Geometry: final body of the model. Coordinates: model frame, mm. A direction names the side the tool comes from. Give positions to 0.01 mm unless a question says otherwise; leave off trailing zeros. Write each loop counter-clockwise with the first axis right and the second up, starting at its lowest first coordinate (ties: lowest second). Pieces come first, ordered by that corner, then holes.
from build123d import *

# Parameters (mm, degrees)
SKETCH1_W           = 29.21
SKETCH1_H           = 35.56
SKETCH1_R           = 1.5499969
BOSS_EXTRUDE1_DEPTH = 5.08
SKETCH2_W           = 5.08
SKETCH2_H           = 25.4
SKETCH2_W_2         = 19.05
SKETCH2_H_2         = 5.08
CUT_EXTRUDE1_DEPTH  = 3.81


with BuildPart() as part:
    # Sketch1 → Boss-Extrude1 (new body)
    with BuildSketch(Plane(origin=(0, 0, 0), x_dir=(1, 0, 0), z_dir=(0, 1, 0))):
        with Locations((2.211294118, -3.505162647)):
            Rectangle(SKETCH1_W, SKETCH1_H)
        with Locations(Location((-9.788707282, 11.694832353, 0), (0, 0, 270))):
            Circle(SKETCH1_R, mode=Mode.SUBTRACT)
        with Locations(Location((14.211295518, 11.694832353, 0), (0, 0, 270))):
            Circle(SKETCH1_R, mode=Mode.SUBTRACT)
        with Locations(Location((14.211295518, -18.705157647, 0), (0, 0, 270))):
            Circle(SKETCH1_R, mode=Mode.SUBTRACT)
        with Locations(Location((-9.788707282, -18.705157647, 0), (0, 0, 270))):
            Circle(SKETCH1_R, mode=Mode.SUBTRACT)
    extrude(amount=BOSS_EXTRUDE1_DEPTH)

    # Sketch2 → Cut-Extrude1 (cut)
    with BuildSketch(Plane(origin=(0, 5.08, 0), x_dir=(1, 0, 0), z_dir=(0, 1, 0))):
        with Locations((-9.853705882, -3.505162647)):
            Rectangle(SKETCH2_W, SKETCH2_H)
        with Locations((2.211294118, 11.734837353)):
            Rectangle(SKETCH2_W_2, SKETCH2_H_2)
        with Locations((14.276294118, -3.505162647)):
            Rectangle(SKETCH2_W, SKETCH2_H)
        with Locations((2.211294118, -3.505162647)):
            Rectangle(SKETCH2_W_2, SKETCH2_H)
        with Locations((2.211294118, -18.745162647)):
            Rectangle(SKETCH2_W_2, SKETCH2_H_2)
    extrude(amount=-CUT_EXTRUDE1_DEPTH, mode=Mode.SUBTRACT)


solid = part.part
Q1. Section D-D on y = 0.5. Output: boundary loops of the cut face in (x, z), plus the area to 3 significant figures.
Filled sheet:
outline: (-12.39, -14.27) - (16.82, -14.27) - (16.82, 21.29) - (-12.39, 21.29) - close; hole circle Ø3.1 at (-9.79, -11.69); hole circle Ø3.1 at (-9.79, 18.71); hole circle Ø3.1 at (14.21, -11.69); hole circle Ø3.1 at (14.21, 18.71)
area: 1,010 mm2
Q2. Pull-direction query (Z, two-part tool) for faces 1 (the cylindrical face through (-9.323, 2.504, 20.184)), 2 (the flat face through (2, 1, -14.275)), 3 (the flat face through (2, 1, 21.285)); classes: released by +Z, released by -Z, zero draft, split by the parting line, or undercut.
Filled sheet:
face 1: undercut
face 2: released by -Z
face 3: released by +Z
Q3. Ray query, line 1 along X through (y, z) = (4.7, 17); line 2 along Z through (x, y) = (-8, 2.85); line 3 along Y through (x, z) = (2.75, -2). Return the intervals inside material, ascending.
Filled sheet:
line 1: x = -12.39 to -7.31, 11.74 to 16.82
line 2: z = -14.27 to -9.19, 16.21 to 21.29
line 3: y = 0 to 1.27
Q4. Section B-B on x = -10.25. Output: boundary loops of the cut face in (y, z).
Filled sheet:
outline: (0, -14.27) - (5.08, -14.27) - (5.08, -13.17) - (0, -13.17) - close; (0, -10.22) - (5.08, -10.22) - (5.08, -9.19) - (1.27, -9.19) - (1.27, 16.21) - (5.08, 16.21) - (5.08, 17.23) - (0, 17.23) - close; (0, 20.18) - (5.08, 20.18) - (5.08, 21.29) - (0, 21.29) - close
Q5. Pin query (flat end, axial travel): P1, Ø4, axis at x = 14.21, z = -11.69, coming from the -Y side; P2, Ø1, axis at x = -4, z = -8.5, coming from the +Y side; P3, Ø3, axis at y = 3, z = -1, coming from the +X side (3 decimals). Return the tip coordinate at first contact, or that it passes through.
Filled sheet:
P1: stops at y = 0
P2: stops at y = 1.27
P3: passes through
Q6. Section C-C on z = -11. Output: boundary loops of the cut face in (x, y), plus the area to 3 significant figures.
Filled sheet:
outline: (-12.39, 0) - (-11.17, 0) - (-11.17, 5.08) - (-12.39, 5.08) - close; (-8.4, 0) - (12.83, 0) - (12.83, 5.08) - (11.74, 5.08) - (11.74, 1.27) - (-7.31, 1.27) - (-7.31, 5.08) - (-8.4, 5.08) - close; (15.6, 0) - (16.82, 0) - (16.82, 5.08) - (15.6, 5.08) - close
area: 47.7 mm2
Q7. Access query for faces 4 (the flat face through (-11, 5.08, -13)), 5 (the flat face through (14, 3, -9.195)), 6 (the flat face through (-7.314, 3, -12)). Directions: +Z, -Z, +X, -X, +Y, -Y. A direction counts if a zero-diameter tool reaches every point of the face in a straight line with its end or side. Return the directions, or none.
Filled sheet:
face 4: +Z, -Z, +X, -X, +Y
face 5: +X, -X, +Y
face 6: +Z, -Z, +Y
Q8. Section A-A on y = 4.55. Output: boundary loops of the cut face in (x, z), plus the area to 3 significant figures.
Filled sheet:
outline: (-12.39, -14.27) - (-7.31, -14.27) - (-7.31, -9.19) - (-12.39, -9.19) - close; (-12.39, 16.21) - (-7.31, 16.21) - (-7.31, 21.29) - (-12.39, 21.29) - close; (11.74, -14.27) - (16.82, -14.27) - (16.82, -9.19) - (11.74, -9.19) - close; (11.74, 16.21) - (16.82, 16.21) - (16.82, 21.29) - (11.74, 21.29) - close; hole circle Ø3.1 at (-9.79, -11.69); hole circle Ø3.1 at (-9.79, 18.71); hole circle Ø3.1 at (14.21, -11.69); hole circle Ø3.1 at (14.21, 18.71)
area: 73.0 mm2
